from build123d import *

# Parameters (mm, degrees)
F0_W     = 36
F0_H     = 18
F1_DEPTH = 3
F2_W     = 30.48
F2_H     = 12
F3_DEPTH = 2
F4_W     = 8
F4_H     = 8
F5_DEPTH = 3.001
F6_R     = 2
F7_R     = 1
F8_DEPTH = 2


with BuildPart() as f1:
    # F0 (on Top) → F1 (new body)
    with BuildSketch(Plane.XY):
        Rectangle(F0_W, F0_H)
    extrude(amount=F1_DEPTH)

    # F2 (on face) → F3 (cut)
    with BuildSketch(Plane.XY.offset(3)):
        Rectangle(F2_W, F2_H)
    extrude(amount=-F3_DEPTH, mode=Mode.SUBTRACT)

    # F4 (on face) → F5 (cut, through all)
    with BuildSketch(Plane(origin=(0, 0, 0), x_dir=(1, 0, 0), z_dir=(0, 0, -1))):
        Rectangle(F4_W, F4_H)
    extrude(amount=-F5_DEPTH, mode=Mode.SUBTRACT)

    # F6
    f6_edges = [f1.edges().sort_by_distance(p)[0] for p in [
        (-18, -9, 1.5),
        (-18, 9, 1.5),
        (18, -9, 1.5),
        (18, 9, 1.5),
    ]]
    fillet(f6_edges, radius=F6_R)

    # F7 (on face) → F8 (cut)
    with BuildSketch(Plane.XY.offset(3)):
        with Locations((-15.24, 6)):
            Circle(F7_R)
        with Locations((-15.24, -6)):
            Circle(F7_R)
        with Locations((15.24, 6)):
            Circle(F7_R)
        with Locations((15.24, -6)):
            Circle(F7_R)
    extrude(amount=-F8_DEPTH, mode=Mode.SUBTRACT)


solid = f1.part
The listing builds one solid part. Answer for the finished solid, in the listing's coordinates (mm). A direction names the side the tool comes from. Give positions to 0.01 mm unless a question says otherwise; leave off trailing zeros. Write each loop counter-clockwise with the first axis right and the second up, starting at its lowest first coordinate (ties: lowest second). Pieces come first, ordered by that corner, then holes. Notation, with made-up numbers: (-24.75, 1) - (-9.75, 1) arc R16 ccw to (-9.75, 13) - close; hole circle Ø7 at (-35, 23.25). An arc over 180 degrees is marked (long way). One line per question, with ' | ' between items. Start each with the question number.
1. Given P1, Ø4, axis at x = -1, y = -3, coming from the +Z side; P2, Ø5, axis at x = -1.5, y = -4.5, coming from the +Z side, each flat-ended and moving along its own axis, determine where each tip first touches the part or whether it passes through.
2. Section D-D, the plane x = -10.5 is taken. Determine the outline of the cut face in (y, z).
3. Determine the mould class of faces 4 (the face through (0, 9, 1)), 5 (the face through (-17.43, 8.4, 1.52)), 6 (the face through (0, -5, 1)) for opening direction X: +X half, -X half, draft (parallel to the pull), parting line (faces both ways), or undercut.
4. Section B-B, the plane x = 3.5 is taken. Determine the outline of the cut face in (y, z).
5. Section C-C, the plane z = 1.4 is taken. Determine the outline of the cut face in (x, y).
6. Section A-A, the plane y = 2 is taken. Determine the outline of the cut face in (x, z), then the cut area to 3 significant figures.
7. For faces 1 (the face through (0, -9, 1)), 2 (the face through (-0.1, -4, 0.5)), 3 (the face through (0, -6, 2)), determine the directions among +Z, -Z, +X, -X, +Y, -Y from which every point of the face is accessible in a straight line to the end or side of a thin tool.
8. Straight lines are drawn through the part: line 1 (X direction, y = 2, z = 2.45); line 2 (Y direction, x = -5, z = 1.55); line 3 (Y direction, x = -15.5, z = 2.6). For each, find the intervals that lie inside material, in ascending order.
Result:
1) P1: stops at z = 1 | P2: stops at z = 3
2) outline: (-9, 0) - (9, 0) - (9, 3) - (6, 3) - (6, 1) - (-6, 1) - (-6, 3) - (-9, 3) - close
3) face 4: draft | face 5: -X half | face 6: undercut
4) outline: (-9, 0) - (-4, 0) - (-4, 1) - (-6, 1) - (-6, 3) - (-9, 3) - close; (4, 0) - (9, 0) - (9, 3) - (6, 3) - (6, 1) - (4, 1) - close
5) outline: (-18, -7) arc R2 ccw to (-16, -9) - (16, -9) arc R2 ccw to (18, -7) - (18, 7) arc R2 ccw to (16, 9) - (-16, 9) arc R2 ccw to (-18, 7) - close; hole (-15.24, -5) arc R1 ccw (long way) to (-14.24, -6) - (14.24, -6) arc R1 ccw (long way) to (15.24, -5) - (15.24, 5) arc R1 ccw (long way) to (14.24, 6) - (-14.24, 6) arc R1 ccw (long way) to (-15.24, 5) - close
6) outline: (-18, 0) - (-4, 0) - (-4, 1) - (-15.24, 1) - (-15.24, 3) - (-18, 3) - close; (4, 0) - (18, 0) - (18, 3) - (15.24, 3) - (15.24, 1) - (4, 1) - close | area: 39.0 mm2
7) face 1: +Z, -Z, +X, -X, -Y | face 2: +Z, -Z | face 3: +Z
8) line 1: x = -18 to -15.24, 15.24 to 18 | line 2: y = -9 to -6, 6 to 9 | line 3: y = -9 to -6.97, -5.03 to 5.03, 6.97 to 9
